from build123d import *

# Parameters (mm, degrees)
F1_DEPTH = 19
F0_W     = 30.2
F0_H     = 14
F2_DEPTH = 4
F3_R     = 2
F4_R     = 3.5
F4_R_2   = 1.725
F5_DEPTH = 2
F6_DEPTH = 4


with BuildPart() as f1:
    # F0 (on Top) → F1 (new body)
    with BuildSketch(Plane.XY):
        Polygon((-4, 0), (0, 0), (0, 14), (30.2, 14), (30.2, 0), (34.2, 0), (34.2, 18), (-4, 18), align=None)
    extrude(amount=F1_DEPTH)

    # F0 (on Top) → F2 (join)
    with BuildSketch(Plane.XY):
        with Locations((15.1, 7)):
            Rectangle(F0_W, F0_H)
        Polygon((-4, 0), (0, 0), (0, 14), (30.2, 14), (30.2, 0), (34.2, 0), (34.2, 18), (-4, 18), align=None)
    extrude(amount=F2_DEPTH)

    # F3
    f3_edges = [f1.edges().sort_by_distance(p)[0] for p in [
        (-4, 18, 9.5),
        (34.2, 18, 9.5),
        (34.2, 0, 9.5),
        (-4, 0, 9.5),
    ]]
    fillet(f3_edges, radius=F3_R)

    # F4 (on face) → F5 (cut)
    with BuildSketch(Plane(origin=(0, 18, 0), x_dir=(-1, 0, 0), z_dir=(0, 1, 0))):
        with Locations((-7.55, 9.5)):
            Circle(F4_R)
        with Locations((-7.55, 9.5)):
            Circle(F4_R_2, mode=Mode.SUBTRACT)
        with Locations((-22.65, 9.5)):
            Circle(F4_R)
        with Locations((-22.65, 9.5)):
            Circle(F4_R_2, mode=Mode.SUBTRACT)
    extrude(amount=-F5_DEPTH, mode=Mode.SUBTRACT)

    # F4 (on face) → F6 (cut, through all)
    with BuildSketch(Plane(origin=(0, 18, 0), x_dir=(-1, 0, 0), z_dir=(0, 1, 0))):
        with Locations((-22.65, 9.5)):
            Circle(F4_R_2)
        with Locations((-7.55, 9.5)):
            Circle(F4_R_2)
    extrude(amount=-F6_DEPTH, mode=Mode.SUBTRACT)


solid = f1.part
The listing builds one solid part. Answer for the finished solid, in the listing's coordinates (mm). A direction names the side the tool comes from. Round coordinates to 2 decimals unless told otherwise and drop trailing zeros. Order: outer loops, then holes, each group sorted by start corner. A loop starts at its lowest first (then second) coordinate and runs counter-clockwise, first axis right, second up. Notation, with made-up numbers: M -25.5,5 L -21.5,5 A19 cw -21.5,33 Z; hole C 29,-14.5 d9. An arc over 180 degrees is marked long. Answer in a Markdown table with one row per item. Add a question column.
1) Which of the six approach directions +Z, -Z, +X, -X, +Y, -Y give full straight-line access (tool end or side, diameter ignored) to faces 4 (the face through (23.409, 17.014, 6.083)), 5 (the face through (33.6, 0.57, 9.63)), 6 (the face through (0, 7, 11))?
2) Flat-ended cylindrical pins translate along their axes: pin 1 Ø4 at (x, y) = (19.5, 10.5) entering from +Z; pin 2 Ø1.5 at (x, z) = (10, 9.5) entering from -Y; pin 3 Ø2 at (x, z) = (8, 8) entering from +Y. Find the tip coordinate at first contact, or state that the pin passes through.
3) The part is cut by section B-B on x = 7.55. Determine the outline of the cut face in (y, z) (3 decimals), plus the area to 3 significant figures.
4) The part is cut by section D-D on z = 5. Determine the outline of the cut face in (x, y).
5) Consider line 1 along Z through (x, y) = (22.65, 15.5) (3 decimals); line 2 along X through (y, z) = (5, 10.5); line 3 along Z through (x, y) = (7.55, 16.8). Determine where each line is inside the solid, lowest interval first. Write a range as from..to.
6) Determine the mould class of faces 1 (the face through (15, 15, 19)), 2 (the face through (15, 7, 4)), 3 (the face through (33.63, 17.4, 9.63)) for opening direction X: pulls with the +X half, pulls with the -X half, needs draft (parallel to the pull), parting line crosses it, or undercut.
7) The part is cut by section A-A on z = 9.5. Determine the outline of the cut face in (x, y) (3 decimals).
8) The part is cut by section C-C on y = 5.25. Determine the outline of the cut face in (x, z), plus the area to 3 significant figures.
Findings below:
| question | item | result |
|---|---|---|
| 1 | face 4 | +Y |
| 1 | face 5 | +Z, -Z, +X, -Y |
| 1 | face 6 | +Z, -Y |
| 2 | pin 1 | stops at z = 4 |
| 2 | pin 2 | stops at y = 14 |
| 2 | pin 3 | stops at y = 16 |
| 3 | outline | M 0,0 L 18,0 L 18,6 L 16,6 L 16,7.775 L 14,7.775 L 14,4 L 0,4 Z; M 14,11.225 L 16,11.225 L 16,13 L 18,13 L 18,19 L 14,19 Z |
| 3 | area | 111 mm² |
| 4 | outline | M -4,2 A2 ccw -2,0 L 0,0 L 0,14 L 30.2,14 L 30.2,0 L 32.2,0 A2 ccw 34.2,2 L 34.2,16 A2 ccw 32.2,18 L -2,18 A2 ccw -4,16 Z |
| 5 | line 1 | z = 0..7.775, 11.225..19 |
| 5 | line 2 | x = -4..0, 30.2..34.2 |
| 5 | line 3 | z = 0..6, 13..19 |
| 6 | face 1 | needs draft |
| 6 | face 2 | undercut |
| 6 | face 3 | pulls with the +X half |
| 7 | outline | M -4,2 A2 ccw -2,0 L 0,0 L 0,14 L 5.825,14 L 5.825,16 L 4.05,16 L 4.05,18 L -2,18 A2 ccw -4,16 Z; M 9.275,14 L 20.925,14 L 20.925,16 L 19.15,16 L 19.15,18 L 11.05,18 L 11.05,16 L 9.275,16 Z; M 24.375,14 L 30.2,14 L 30.2,0 L 32.2,0 A2 ccw 34.2,2 L 34.2,16 A2 ccw 32.2,18 L 26.15,18 L 26.15,16 L 24.375,16 Z |
| 8 | outline | M -4,0 L 34.2,0 L 34.2,19 L 30.2,19 L 30.2,4 L 0,4 L 0,19 L -4,19 Z |
| 8 | area | 273 mm² |
